Autodesk Inventor part; units mm, degrees
ref_plane "工作平面4" through (-13.0444, 62, -10.5556) normal (-0.9848, 0.1736, 0) x (0, 0, 1)
ref_plane "YZ Plane" through (0, 0, 0) normal (1, 0, 0) x (0, 1, 0)
ref_plane "XZ Plane" through (0, 0, 0) normal (0, 1, 0) x (-1, 0, 0)
sketch "草图1" plane through (0, 0, 0) normal (0, 1, 0) x (-1, 0, 0)
  line L0 (20.0444, 13.4444) -> (-9.9556, 13.4444)
  line L1 (-9.9556, 13.4444) -> (-9.9556, -16.5556)
  line L2 (-9.9556, -16.5556) -> (20.0444, -16.5556)
  line L3 (20.0444, -16.5556) -> (20.0444, 13.4444)
  line L4 (0.0444, 13.4444) -> (-7.4556, 13.4444)
  line L5 (0.0444, 13.4444) -> (7.5444, 13.4444)
  dimension "d0" = 30
  dimension "d1" = 30
extrude "拉伸1" add sketch "草图1" along normal blind 2
sketch "草图2" plane through (0, 2, 0) normal (0, 1, 0) x (1, 0, 0)
  line L0 (9.9556, 16.5556) -> (-20.0444, 16.5556)
  circle A0 centre (4.9556, 12.5556) radius 1.5
  circle A1 centre (-10.0444, 12.5556) radius 1.5
  circle A2 centre (-10.0444, -9.4444) radius 1.5
  circle A3 centre (4.9556, -9.4444) radius 1.5
  line L1 (-10.0444, 12.5556) -> (-10.0444, 16.5556)
  line L2 (4.9556, 12.5556) -> (4.9556, 16.5556)
  line L3 (-10.0444, -9.4444) -> (-10.0444, -13.4444)
  line L4 (-20.0444, -13.4444) -> (9.9556, -13.4444)
  line L5 (4.9556, -9.4444) -> (4.9556, -13.4444)
  line L6 (9.9556, -13.4444) -> (9.9556, 16.5556)
  line L7 (-20.0444, 16.5556) -> (-20.0444, -13.4444)
  point P0 (0, 0)
  dimension "d15" = 3
  dimension "d16" = 3
  dimension "d17" = 3
  dimension "d108" = 4
  dimension "d109" = 4
  dimension "d110" = 4
  dimension "d111" = 4
  dimension "d112" = 5
  dimension "d113" = 10
extrude "拉伸2" cut sketch "草图2" against normal blind 2 contours A0 | A1 | A2 | A3
sketch "草图3" plane through (0, 2, 0) normal (0, 1, 0) x (1, 0, 0)
  circle A0 centre (4.9556, 12.5556) radius 1.5
  circle A1 centre (-10.0444, -9.4444) radius 1.5
  line L0 (2.9556, 10.5556) -> (2.9556, -7.4444)
  line L1 (-13.0444, 10.5556) -> (-13.0444, -7.4444)
  line L2 (-13.0444, -7.4444) -> (2.9556, -7.4444)
  line L3 (-13.0444, 10.5556) -> (2.9556, 10.5556)
  line L4 (-22.598, 1.5556) -> (13.9828, 1.5556)
  point P0 (0, 0)
  dimension "d137" = 11
extrude "拉伸3" add sketch "草图3" along normal blind 60 contours L0 L4 L1 L3 | L0 L2 L1 L4
chamfer "倒角5" distance 16 angle 10 1 edges at (2.9556, 62, -1.5556) measured on face at (-2.3778, 62, 1.4444)
sketch "草图29" plane through (0, 2, 0) normal (0, 1, 0) x (1, 0, 0)
  line L0 (-13.0444, -7.4444) -> (-13.0444, 10.5556)
  line L1 (-13.0444, 10.5556) -> (-20.9964, 10.5556)
  line L2 (-20.9964, 10.5556) -> (-20.9964, -16.1821)
  line L3 (-20.9964, -16.1821) -> (-13.0444, -16.1821)
  line L4 (-13.0444, -16.1821) -> (-13.0444, 10.5556)
  line L5 (-13.0444, 10.5556) -> (-22.8537, 10.5556)
  line L6 (-22.8537, 10.5556) -> (-22.8537, 28.4787)
  line L7 (-22.8537, 28.4787) -> (-13.0444, 28.4787)
  line L8 (-13.0444, 28.4787) -> (-13.0444, 10.5556)
  point P0 (0, 0)
  point P1 (-20.0444, -13.4444)
extrude "拉伸15" cut sketch "草图29" against normal blind 20
sketch "草图31" plane through (-13.0444, 62, 7.4444) normal (0.1736, 0.9848, 0) x (0.9848, -0.1736, 0)
  line L0 (0, 18) -> (0, 0)
  line L1 (0, 9) -> (16.2468, 9)
  line L2 (16.2468, 0) -> (16.2468, 18)
  circle A0 centre (8.1234, 9) radius 1.5
  point P0 (23.6125, 7.4444)
  dimension "d134" = 3
extrude "拉伸16" cut sketch "草图31" against normal blind 20
ref_plane "工作平面4" through (-13.0444, 62, -10.5556) normal (-0.9848, 0.1736, 0) x (0, 0, 1)
ref_plane "工作平面3" through (2.9556, 59.1788, -1.5556) normal (0.1736, 0.9848, 0) x (0.9848, -0.1736, 0)
sketch "草图36" plane through (-13.0444, 62, -10.5556) normal (-0.9848, 0.1736, 0) x (0, 0, 1)
  line L0 (18, 0) -> (0, 0)
  circle A0 centre (9, 0) radius 15
  point P0 (10.5556, -58.7929)
  dimension "d140" = 30
extrude "拉伸17" cut sketch "草图36" against normal blind 200
sketch "草图38" plane through (-13.0444, 62, -10.5556) normal (-0.9848, 0.1736, 0) x (0, 0, 1)
  line L0 (9, -17.5895) -> (9, 63.4105)
  circle A0 centre (9, 22.9105) radius 40.5
  point P0 (10.5556, -58.7929)
  dimension "d143" = 81
extrude "拉伸18" add sketch "草图38" against normal blind 20
sketch "草图39" plane through (-9.0661, 84.5624, -1.5556) normal (-0.9848, 0.1736, 0) x (0, 0, 1)
  line L0 (-48.0605, 0) -> (68.7188, 0)
  line L1 (68.7188, 0) -> (68.7188, 57.1611)
  line L2 (68.7188, 57.1611) -> (-48.0605, 57.1611)
  line L3 (-48.0605, 57.1611) -> (-48.0605, 0)
  point P0 (1.5556, -81.7034)
extrude "拉伸19" cut sketch "草图39" against normal through all
sketch "草图41" plane through (-13.0444, 62, -10.5556) normal (-0.9848, 0.1736, 0) x (0, 0, 1)
  line L0 (49.5, 22.9105) -> (-31.5, 22.9105)
  circle A0 centre (9, 22.9105) radius 40
  point P0 (10.5556, -58.7929)
  dimension "d148" = 80
extrude "拉伸20" cut sketch "草图41" against normal blind 20
equation "\"折弯半径\" = 厚度"
equation "\"折弯释压宽度\" = 厚度"
equation "\"折弯释压深度\" = 0.5 * 厚度"
equation "\"拐角释压尺寸\" = 4 * 厚度"
equation "\"最小余量\" = 2 * 厚度"
equation "\"过渡半径\" = 折弯半径"
equation "\"Jacobi半径尺寸\" = 折弯半径"
equation "\"间隙大小\" = 厚度"
properties part number "_3D 打印"
Check sheet for the modelled part. Datum: model origin and axes. Units: mm. A direction names the side the tool comes from. Round coordinates to 2 decimals unless told otherwise and drop trailing zeros. Order: outer loops, then holes, each group sorted by start corner. A loop starts at its lowest first (then second) coordinate and runs counter-clockwise, first axis right, second up.
1) Scan lines: line 1 (Z direction, x = -6, y = 14); line 2 (Y direction, x = 6.75, z = -15.5); line 3 (Z direction, x = -7.5, y = 59.5). Record each from-to range of solid material in increasing order.
2) Mould release check, pull along Y, two halves, no side actions. Record for faces 4 (the flat face through (-5, 23, 7.444)), 5 (the flat face through (0.64, 82.85, -41.81)), 6 (the flat face through (-1, 1, -16.556)): +Y half, -Y half, draft (parallel to the pull), parting line (faces both ways), or undercut.
3) Section check B-B (z = 2.5). Record the boundary of the cut face in (x, y).
4) Tool access check on faces 1 (the flat face through (-2, 1, 13.444)), 2 (the cylindrical face through (4.76, 1.014, 7.957)), 3 (the flat face through (-8.538, 40.895, -1.577)). Record the directions out of +Z, -Z, +X, -X, +Y, -Y that give a thin tool (end or side, any length) a straight path to the whole face; none if there is none.
5) Go/stop test with flat-tipped pins: pin 1 Ø5 at (y, z) = (43, -12) entering from +X; pin 2 Ø4 at (x, y) = (-0.5, 37.5) entering from -Z; pin 3 Ø3.5 at (x, z) = (-10.04, -12.56) entering from +Y; pin 4 Ø2 at (x, z) = (6, 14.5) entering from +Y. Record where each tip stops, or that it passes through.
6) Section check C-C (z = -9). Record the boundary of the cut face in (x, y), and give its area (3 significant figures).
7) Section check D-D (z = 16.5). Record the boundary of the cut face in (x, y).
8) Section check A-A (y = 26). Record the boundary of the cut face in (x, z), and give its area (3 significant figures).
Result:
1. line 1: z = -10.56 to 7.44
1. line 2: y = 0 to 2
1. line 3: z = -33.87 to -33.24, 30.13 to 30.76
2. face 4: undercut
2. face 5: +Y half
2. face 6: draft
3. outline: (-16.06, 44.88) - (-13.04, 44.35) - (-13.04, 0) - (9.96, 0) - (9.96, 2) - (2.96, 2) - (2.96, 41.52) - (3.63, 41.41) - (3.72, 41.9) - (-15.98, 45.37) - close
4. face 1: +Z, +X, -X, -Y
4. face 2: -Y
4. face 3: none
5. pin 1: stops at x = 4.05
5. pin 2: stops at z = -10.56
5. pin 3: stops at y = 46.31
5. pin 4: passes through
6. outline: (-15.98, 45.36) - (-13.04, 44.84) - (-13.04, 0) - (9.96, 0) - (9.96, 2) - (2.96, 2) - (2.96, 42.02) - (3.72, 41.88) - (3.81, 42.39) - (-15.89, 45.86) - close
6. area: 719 mm2
7. outline: (-15.36, 48.86) - (4.33, 45.39) - (4.43, 45.94) - (-15.26, 49.41) - close
8. outline: (-13.04, -10.56) - (2.96, -10.56) - (2.96, 7.44) - (-13.04, 7.44) - close
8. area: 288 mm2
